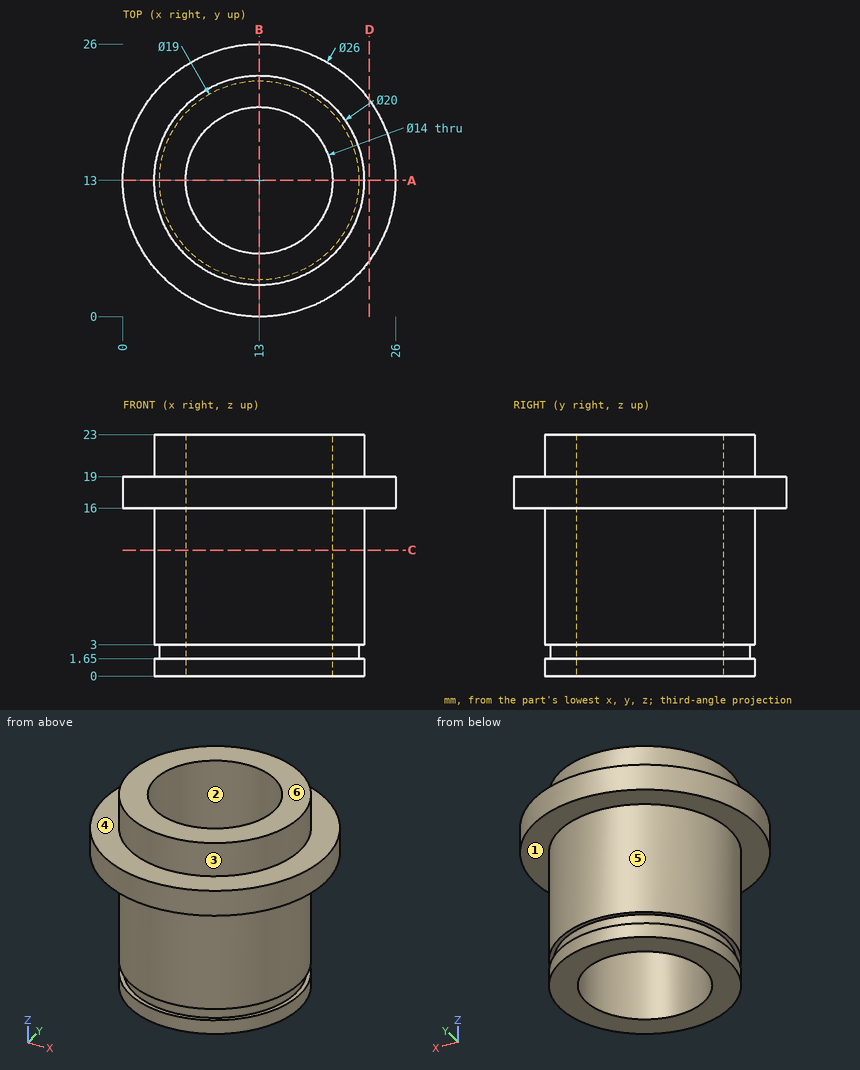
Geometry: see drawing. Coordinates: mm, zero at the bounding-box minimum. A direction names the side the tool comes from. Round coordinates to 2 decimals unless told otherwise and drop trailing zeros. Write each loop counter-clockwise with the first axis right and the second up, starting at its lowest first coordinate (ties: lowest second). Pieces come first, ordered by that corner, then holes.
1) Reachability of the marked faces 4, 5 and 6 from +Z, -Z, +X, -X, +Y, -Y: full face, straight path, thin tool, end or side. Return the list, or none.
2) Draft query along X for the marked faces 1, 2 and 3. Return one class per face: pulls with the +X half, pulls with the -X half, needs draft (parallel to the pull), parting line crosses it, or undercut.
3) Cut plane D-D (x = 23.5). Return the cut outline in (y, z).
4) Cut plane C-C (z = 12). Return the cut outline in (x, y), then the cut area to 3 significant figures.
5) Ray query, L1, parallel to Y at x = 13, z = 17.75; L2, parallel to Z at x = 21, y = 18.75; L3, parallel to Y at x = 13, z = 11. Return the intervals inside material, ascending.
6) Cut plane A-A (y = 13). Return the cut outline in (x, z), then the cut area to 3 significant figures.
7) Contact query for flat-ended pins moving along their axis: P1, Ø2, axis at x = 22, z = 4.5, coming from the +Y side; P2, Ø1.5, axis at y = 15.5, z = 4.5, coming from the -X side; P3, Ø1.5, axis at x = 22, y = 5, coming from the +Z side. Output: stop coordinate, or through.
Geometry says:
1. face 4: +Z
1. face 5: -Z
1. face 6: +Z, +X, -X, +Y, -Y
2. face 1: needs draft
2. face 2: undercut
2. face 3: parting line crosses it
3. outline: (5.34, 16) - (20.66, 16) - (20.66, 19) - (5.34, 19) - close
4. outline: circle Ø20 at (13, 13); hole circle Ø14 at (13, 13)
4. area: 160 mm2
5. L1: y = 0 to 6, 20 to 26
5. L2: z = 0 to 1.65, 3 to 23
5. L3: y = 3 to 6, 20 to 23
6. outline: (0, 16) - (3, 16) - (3, 3) - (3.5, 3) - (3.5, 1.65) - (3, 1.65) - (3, 0) - (6, 0) - (6, 23) - (3, 23) - (3, 19) - (0, 19) - close; (20, 0) - (23, 0) - (23, 1.65) - (22.5, 1.65) - (22.5, 3) - (23, 3) - (23, 16) - (26, 16) - (26, 19) - (23, 19) - (23, 23) - (20, 23) - close
6. area: 155 mm2
7. P1: stops at y = 19
7. P2: stops at x = 3.15
7. P3: stops at z = 19
